Could you check a few things on this model? Use its own coordinates, in mm. Give positions to 0.01 mm unless a question says otherwise; leave off trailing zeros. Write each loop counter-clockwise with the first axis right and the second up, starting at its lowest first coordinate (ties: lowest second). Pieces come first, ordered by that corner, then holes. Notation, with made-up numbers: (74.5, 39.5) - (95.5, 39.5) arc R19 cw to (95.5, 67.5) - close; hole circle Ø8 at (22, 61). An arc over 180 degrees is marked (long way). Answer in a Markdown table with one row per item.
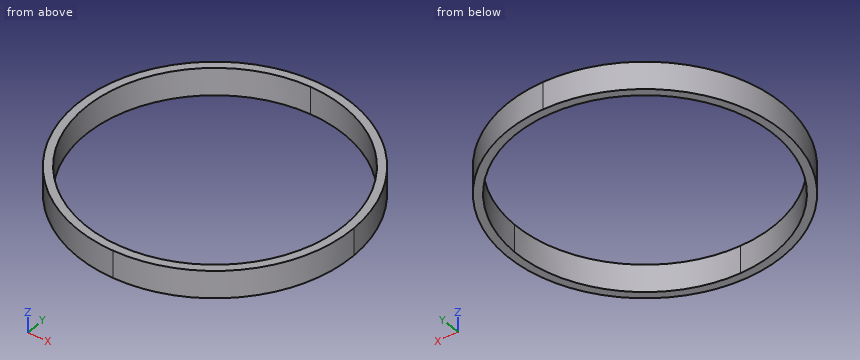
from build123d import *

# Parameters (mm, degrees)
F1_DEPTH = 31.75


with BuildPart() as f1:
    # F0 (on Top) → F1 (new body)
    with BuildSketch(Plane.XY):
        with BuildLine():
            ThreePointArc((0, -158.623), (112.163399, -112.163399), (158.623, 0))
            ThreePointArc((158.623, 0), (112.163399, 112.163399), (0, 158.623))
            Line((0, 158.623), (0, 149.225))
            ThreePointArc((0, 149.225), (105.518009, 105.518009), (149.225, 0))
            ThreePointArc((149.225, 0), (105.518009, -105.518009), (0, -149.225))
            Line((0, -149.225), (0, -158.623))
        make_face()
        with BuildLine():
            Line((0, 149.225), (0, 158.623))
            ThreePointArc((0, 158.623), (-158.623, 0), (0, -158.623))
            Line((0, -158.623), (0, -149.225))
            ThreePointArc((0, -149.225), (-149.225, 0), (0, 149.225))
        make_face()
    extrude(amount=F1_DEPTH)


solid = f1.part
1) Imagine slicing it at A-A (y = 39). List the corners of the cut face in (x, z) for me.
Check values:
| item | result |
|---|---|
| outline | (-153.75, 0) - (-144.04, 0) - (-144.04, 31.75) - (-153.75, 31.75) - close; (144.04, 0) - (153.75, 0) - (153.75, 31.75) - (144.04, 31.75) - close |
2) If I drill on line 1 (Y direction, x = 38, z = 7.5); line 2 (Y direction, x = 59.5, z = 21); line 3 (X direction, y = -129, z = 30.5), over which ranges is the centre line in solid material (lowest first)?
Check values:
| item | result |
|---|---|
| line 1 | y = -154 to -144.31, 144.31 to 154 |
| line 2 | y = -147.04 to -136.85, 136.85 to 147.04 |
| line 3 | x = -92.31 to -75.01, 75.01 to 92.31 |
3) Will these pins go through, and if not, where does the flat tip stop? P1, Ø3, axis at y = 89.5, z = 13.5, coming from the -X side; P2, Ø1, axis at x = -26, z = 21.5, coming from the +Y side; P3, Ø4, axis at x = 27.5, z = 10, coming from the -Y side.
Check values:
| item | result |
|---|---|
| P1 | stops at x = -131.97 |
| P2 | stops at y = 156.56 |
| P3 | stops at y = -156.56 |
4) Imagine slicing it at C-C (z = 14.5). List the corners of the cut face in (x, y) for me (3 decimals), then the cut area to 3 significant figures.
Check values:
| item | result |
|---|---|
| outline | circle Ø317.246 at (0, 0); hole (0, -149.225) arc R149.225 ccw to (149.225, 0) arc R149.225 ccw to (0, 149.225) arc R149.225 ccw to start |
| area | 9,090 mm2 |
5) Imagine slicing it at B-B (x = -61). List the corners of the cut face in (y, z) for me, then the cut area to 3 significant figures.
Check values:
| item | result |
|---|---|
| outline | (-146.42, 0) - (-136.19, 0) - (-136.19, 31.75) - (-146.42, 31.75) - close; (136.19, 0) - (146.42, 0) - (146.42, 31.75) - (136.19, 31.75) - close |
| area | 650 mm2 |
